```python
from build123d import *

# Parameters (mm, degrees)
SKETCH1_R           = 19.05
BOSS_EXTRUDE1_DEPTH = 16
SKETCH2_R           = 15.4
CUT_EXTRUDE1_DEPTH  = 10
SKETCH4_R           = 2.5
CUT_EXTRUDE3_DEPTH  = 1.4
SKETCH5_R           = 1.4
CUT_EXTRUDE4_DEPTH  = 5.6
SKETCH6_R           = 1.4
CUT_EXTRUDE5_DEPTH  = 5.6
SKETCH9_R           = 1.4
CUT_EXTRUDE8_DEPTH  = 5.6
SKETCH10_R          = 1.4
CUT_EXTRUDE9_DEPTH  = 5.6
SKETCH11_R          = 6
CUT_EXTRUDE11_DEPTH = 7


with BuildPart() as part:
    # Sketch1 → Boss-Extrude1 (new body)
    with BuildSketch(Plane.XY):
        Circle(SKETCH1_R)
    extrude(amount=BOSS_EXTRUDE1_DEPTH)

    # Sketch2 → Cut-Extrude1 (cut)
    with BuildSketch(Plane(origin=(0, 0, 0), x_dir=(-1, 0, 0), z_dir=(0, 0, -1))):
        Circle(SKETCH2_R)
    extrude(amount=-CUT_EXTRUDE1_DEPTH, mode=Mode.SUBTRACT)

    # Sketch4 → Cut-Extrude3 (cut)
    with BuildSketch(Plane(origin=(0, 0, 10), x_dir=(-1, 0, 0), z_dir=(0, 0, -1))):
        with Locations((-7, 7)):
            Circle(SKETCH4_R)
        with Locations((7, 7)):
            Circle(SKETCH4_R)
        with Locations((7, -7)):
            Circle(SKETCH4_R)
        with Locations((-7, -7)):
            Circle(SKETCH4_R)
    extrude(amount=-CUT_EXTRUDE3_DEPTH, mode=Mode.SUBTRACT)

    # Sketch5 → Cut-Extrude4 (cut, through all)
    with BuildSketch(Plane(origin=(0, 0, 11.4), x_dir=(-1, 0, 0), z_dir=(0, 0, -1))):
        with Locations((-6.998002378, 7.019977132)):
            Circle(SKETCH5_R)
    extrude(amount=-CUT_EXTRUDE4_DEPTH, mode=Mode.SUBTRACT)

    # Sketch6 → Cut-Extrude5 (cut, through all)
    with BuildSketch(Plane(origin=(0, 0, 11.4), x_dir=(-1, 0, 0), z_dir=(0, 0, -1))):
        with Locations((7.062657108, 6.986426582)):
            Circle(SKETCH6_R)
    extrude(amount=-CUT_EXTRUDE5_DEPTH, mode=Mode.SUBTRACT)

    # Sketch9 → Cut-Extrude8 (cut, through all)
    with BuildSketch(Plane(origin=(0, 0, 11.4), x_dir=(-1, 0, 0), z_dir=(0, 0, -1))):
        with Locations((-7, -7)):
            Circle(SKETCH9_R)
    extrude(amount=-CUT_EXTRUDE8_DEPTH, mode=Mode.SUBTRACT)

    # Sketch10 → Cut-Extrude9 (cut, through all)
    with BuildSketch(Plane(origin=(0, 0, 11.4), x_dir=(-1, 0, 0), z_dir=(0, 0, -1))):
        with Locations((7, -7)):
            Circle(SKETCH10_R)
    extrude(amount=-CUT_EXTRUDE9_DEPTH, mode=Mode.SUBTRACT)

    # Sketch11 → Cut-Extrude11 (cut, through all)
    with BuildSketch(Plane(origin=(0, 0, 10), x_dir=(-1, 0, 0), z_dir=(0, 0, -1))):
        Circle(SKETCH11_R)
    extrude(amount=-CUT_EXTRUDE11_DEPTH, mode=Mode.SUBTRACT)


solid = part.part
```
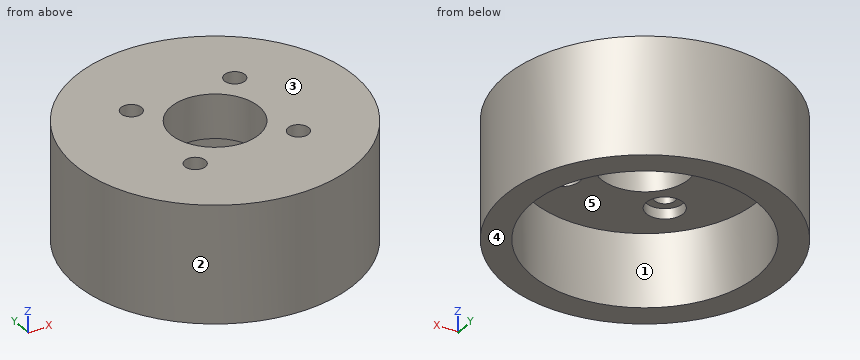
Model file for the job. Use its own axes, mm. Face numbers are marked on the shaded views. A direction names the side the tool comes from. Coordinates: 2 decimals unless noted, no trailing zeros. Order: outer loops, then holes, each group sorted by start corner. A loop starts at its lowest first (then second) coordinate and runs counter-clockwise, first axis right, second up. Notation, with made-up numbers: (39, 23.25) -> (46, 23.25) arc R16 ccw to (46, 41.25) -> close; hole circle Ø9 at (-2, 32.5). An arc over 180 degrees is marked (long way). Return JSON: item names as keys, results as strings.
Item 1: Mould opens along Y. For the marked faces 1, 2 and 3 say: pulls with the +Y half, pulls with the -Y half, needs draft (parallel to the pull), parting line crosses it, or undercut.
Model answer:
{"face 1": "undercut", "face 2": "parting line crosses it", "face 3": "needs draft"}
Item 2: Slice it at D-D (z = 5). Write the cut outline in (x, y), then the cut area to 3 significant figures.
Model answer:
{"outline": "circle Ø38.1 at (0, 0); hole circle Ø30.8 at (0, 0)", "area": "395 mm²"}
Item 3: 3-axis set-ups, long thin cutter, end or side, ignore diameter. For the marked faces 4 and 5: which of +Z, -Z, +X, -X, +Y, -Y reach the whole face in a straight line?
Model answer:
{"face 4": "-Z, +X, -X, +Y, -Y", "face 5": "-Z"}
Item 4: Pin check, flat tips, straight feed: P1, Ø5.5, axis at x = 8, y = -6.5, coming from the -Z side; P2, Ø1, axis at y = -15, z = 4, coming from the +X side; P3, Ø1.5, axis at x = -12, z = 4.5, coming from the -Y side. Stop position of each tip, or through.
Model answer:
{"P1": "stops at z = 10", "P2": "stops at x = 12.36", "P3": "stops at y = -15.37"}
Item 5: Wall check: line 1 along Y through (x, z) = (7, 10.95); line 2 along Y through (x, z) = (0, 7); line 3 along X through (y, z) = (-7.5, 14.5). Give the ranges that are in metal, low to high. Write a range as from..to.
Model answer:
{"line 1": "y = -17.72..-9.5, -4.5..4.5, 9.5..17.72", "line 2": "y = -19.05..-15.4, 15.4..19.05", "line 3": "x = -17.51..-8.31, -5.69..5.69, 8.31..17.51"}
Item 6: Slice it at B-B (y = 7.5). Write the cut outline in (x, z), then the cut area to 3 significant figures.
Model answer:
{"outline": "(-17.51, 0) -> (-13.45, 0) -> (-13.45, 10) -> (-9.45, 10) -> (-9.45, 11.4) -> (-8.37, 11.4) -> (-8.37, 16) -> (-17.51, 16) -> close; (-5.76, 11.4) -> (-4.55, 11.4) -> (-4.55, 10) -> (4.55, 10) -> (4.55, 11.4) -> (5.68, 11.4) -> (5.68, 16) -> (-5.76, 16) -> close; (8.31, 11.4) -> (9.45, 11.4) -> (9.45, 10) -> (13.45, 10) -> (13.45, 0) -> (17.51, 0) -> (17.51, 16) -> (8.31, 16) -> close", "area": "254 mm²"}
Item 7: Slice it at A-A (y = 0). Write the cut outline in (x, z), then the cut area to 3 significant figures.
Model answer:
{"outline": "(-19.05, 0) -> (-15.4, 0) -> (-15.4, 10) -> (-6, 10) -> (-6, 16) -> (-19.05, 16) -> close; (6, 10) -> (15.4, 10) -> (15.4, 0) -> (19.05, 0) -> (19.05, 16) -> (6, 16) -> close", "area": "230 mm²"}
Item 8: Slice it at C-C (x = 7). Write the cut outline in (y, z).
Model answer:
{"outline": "(-17.72, 0) -> (-13.72, 0) -> (-13.72, 10) -> (-9.5, 10) -> (-9.5, 11.4) -> (-8.4, 11.4) -> (-8.4, 16) -> (-17.72, 16) -> close; (-5.6, 11.4) -> (-4.5, 11.4) -> (-4.5, 10) -> (4.5, 10) -> (4.5, 11.4) -> (5.62, 11.4) -> (5.62, 16) -> (-5.6, 16) -> close; (8.42, 11.4) -> (9.5, 11.4) -> (9.5, 10) -> (13.72, 10) -> (13.72, 0) -> (17.72, 0) -> (17.72, 16) -> (8.42, 16) -> close"}
